Model file for the job. Use its own axes, mm. Face numbers are marked on the shaded views. A direction names the side the tool comes from. Coordinates: 2 decimals unless noted, no trailing zeros. Order: outer loops, then holes, each group sorted by start corner. A loop starts at its lowest first (then second) coordinate and runs counter-clockwise, first axis right, second up. Notation, with made-up numbers: (67.5, -27.5) -> (77.5, -27.5) arc R20 ccw to (77.5, -1.5) -> close; hole circle Ø9 at (60, 20.25). An arc over 180 degrees is marked (long way). Use CSV: the item, a comma, the result in double quotes. Start each with the question number.
(1) Cut at C-C on z = -51.5. Write the cut outline in (x, y).
(2) Pull direction Y, two halves, no side cores. Call the marked faces 1, 2, 3 and 4: pulls with the +Y half, pulls with the -Y half, needs draft (parallel to the pull), parting line crosses it, or undercut.
(3) Cut at D-D on y = 64.5. Write the cut outline in (x, z).
(4) Tool access for the marked faces 5 and 6: list every direction of +Z, -Z, +X, -X, +Y, -Y with a clear straight run to the whole face (end or side of a thin tool).
(5) Pin check, flat tips, straight feed: pin 1 Ø1.5 at (x, y) = (198, 21.5) entering from +Z; pin 2 Ø5 at (x, y) = (171.5, 54.5) entering from +Z; pin 3 Ø1.5 at (x, y) = (57, 48) entering from -Z. Stop position of each tip, or through.
(6) Cut at B-B on y = 50. Give the number of separate pieces and of enclosed holes in the cut face, plus the area to 3 significant figures.
(7) Probe L1, parallel to Y at x = 168, z = -37; L2, parallel to X at y = 78.5, z = -75.5; L3, parallel to Y at x = 9, z = -64.5. List the from-to ranges inside material, lowest first.
Autodesk Inventor part; units mm, degrees
ref_plane "YZ Plane" through (0, 0, 0) normal (1, 0, 0) x (0, 1, 0)
ref_plane "XZ Plane" through (0, 0, 0) normal (0, 1, 0) x (-1, 0, 0)
ref_plane "XY Plane" through (0, 0, 0) normal (0, 0, 1) x (1, 0, 0)
sketch "Sketch1" plane through (0, 0, 0) normal (0, 0, 1) x (1, 0, 0)
  line L0 (0, 0) -> (200, 0)
  line L1 (200, 0) -> (200, 90)
  line L2 (200, 90) -> (0, 90)
  line L3 (0, 90) -> (0, 0)
  dimension "d0" = 200
  dimension "d1" = 90
extrude "Extrusion1" add sketch "Sketch1" against normal blind 80
sketch "Sketch2" plane through (0, 90, 0) normal (0, 1, 0) x (1, 0, 0)
  line L0 (200, 0) -> (0, 0)
  line L1 (200, 0) -> (200, 80)
  line L2 (0, 80) -> (200, 80)
  line L3 (0, 0) -> (0, 80)
  circle A0 centre (100, 0) radius 30
  arc A1 (200, 0) -> (0, 0) centre (100, -151.6667) ccw
  dimension "d4" = 60
extrude "Extrusion2" cut sketch "Sketch2" against normal blind 100 contours L0 A0 A1 | L0 A0 | A0 L0 A1 picked at (94.9216, 15.5737)
fillet "Fillet1" radius 15 2 edges at (200, 45, 0) (0, 45, 0)
sketch "Sketch3" plane through (200, 0, -80) normal (1, 0, 0) x (0, 0, -1)
  line L0 (-80, 0) -> (-80, 90)
  line L1 (-80, 0) -> (0, 0)
  line L2 (0, 90) -> (0, 0)
  line L3 (-80, 90) -> (0, 90)
  line L4 (-12, 25) -> (-11.3, 25)
  line L5 (-10, 23.7) -> (-10, 16.3)
  line L6 (-11.3, 15) -> (-12, 15)
  line L7 (-13.3, 16.3) -> (-13.3, 23.7)
  arc A0 (-12, 25) -> (-13.3, 23.7) centre (-12, 23.7) ccw
  arc A1 (-10, 23.7) -> (-11.3, 25) centre (-11.3, 23.7) ccw
  arc A2 (-11.3, 15) -> (-10, 16.3) centre (-11.3, 16.3) ccw
  arc A3 (-13.3, 16.3) -> (-12, 15) centre (-12, 16.3) ccw
  point P0 (-10, 15)
  point P1 (-10, 25)
  point P2 (-13.3, 15)
  point P3 (-11.65, 15)
  dimension "d8" = 3.3
  dimension "d9" = 10
  dimension "d10" = 1.3
  dimension "d11" = 10
  dimension "d12" = 15
fillet "Fillet3" radius 10 10 edges at (7.0077, 0, -12.9892) (0, 0, -52.8413) (192.9923, 0, -12.9892) (200, 0, -52.8413) (100, 0, -30) (192.9923, 90, -12.9892) (200, 90, -52.8413) (7.0077, 90, -12.9892) (0, 90, -52.8413) (100, 90, -30)
shell "Shell2" thickness 5 removed faces 1 at (130, 30, -80)
extrude "Extrusion4" cut sketch "Sketch3" against normal blind 100 contours L4 A1 L5 A2 L6 A3 L7 A0
fillet "Fillet4" radius 1 16 edges at (200, 24.6192, -67.0808) (200, 25, -68.35) (200, 24.6192, -69.6192) (200, 20, -70) (200, 15.3808, -69.6192) (200, 15, -68.35) (200, 15.3808, -67.0808) (200, 20, -66.7) (195, 15.3808, -67.0808) (195, 15, -68.35) (195, 15.3808, -69.6192) (195, 20, -70) (195, 24.6192, -69.6192) (195, 25, -68.35) (195, 24.6192, -67.0808) (195, 20, -66.7)
sketch "Sketch6" plane through (200, 10, -25.6826) normal (1, 0, 0) x (0, 0, -1)
  line L0 (0, 70) -> (54.3174, 70)
  line L1 (0, 0) -> (0, 70)
  line L2 (54.3174, 0) -> (0, 0)
  line L3 (54.3174, 70) -> (54.3174, 0)
  arc A0 (42.3174, 16) -> (40.0174, 13.7) centre (42.3174, 13.7) ccw
  line L4 (43.0174, 16) -> (42.3174, 16)
  arc A1 (45.3174, 13.7) -> (43.0174, 16) centre (43.0174, 13.7) ccw
  line L5 (45.3174, 6.3) -> (45.3174, 13.7)
  arc A2 (43.0174, 4) -> (45.3174, 6.3) centre (43.0174, 6.3) ccw
  line L6 (42.3174, 4) -> (43.0174, 4)
  arc A3 (40.0174, 6.3) -> (42.3174, 4) centre (42.3174, 6.3) ccw
  line L7 (40.0174, 13.7) -> (40.0174, 6.3)
  line L8 (44.3174, 42.5) -> (34.3174, 42.5)
  line L9 (34.3174, 42.5) -> (34.3174, 27.5)
  line L10 (34.3174, 27.5) -> (44.3174, 27.5)
  line L11 (44.3174, 27.5) -> (44.3174, 42.5)
  point P0 (-25.6826, -10)
  point P1 (44.3174, 35)
  point P2 (54.3174, 35)
  dimension "d32" = 10
  dimension "d33" = 15
  dimension "d34" = 10
extrude "Extrusion7" cut sketch "Sketch6" against normal blind 5 contours L11 L10 L9 L8
sketch "Sketch7" plane through (0, 10, -80) normal (-1, 0, 0) x (0, 0, 1)
  line L0 (0, 70) -> (54.3174, 70)
  line L1 (0, 0) -> (0, 70)
  line L2 (54.3174, 0) -> (0, 0)
  line L3 (54.3174, 70) -> (54.3174, 0)
  line L4 (10, 42.5) -> (20, 42.5)
  line L5 (20, 42.5) -> (20, 27.5)
  line L6 (20, 27.5) -> (10, 27.5)
  line L7 (10, 27.5) -> (10, 42.5)
  point P0 (80, -10)
  point P1 (10, 35)
  point P2 (0, 35)
  dimension "d37" = 10
  dimension "d38" = 15
  dimension "d39" = 10
extrude "Extrusion8" cut sketch "Sketch7" against normal blind 5 contours L4 L5 L6 L7
fillet "Fillet5" radius 2.5 12 edges at (195, 45, -60) (195, 52.5, -65) (195, 37.5, -65) (200, 45, -60) (200, 37.5, -65) (200, 52.5, -65) (0, 45, -60) (5, 45, -60) (5, 52.5, -65) (0, 52.5, -65) (0, 37.5, -65) (5, 37.5, -65)
properties part number "BatPackCase_3DPrint"
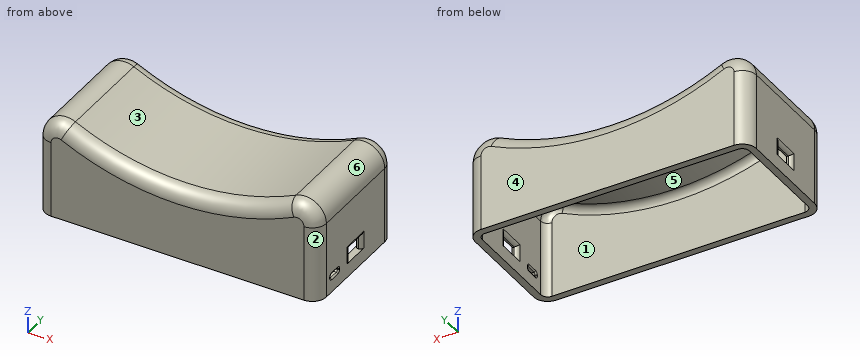
Outcome:
1,outline,"(0, 10) arc R10 ccw to (10, 0) -> (190, 0) arc R10 ccw to (200, 10) -> (200, 80) arc R10 ccw to (190, 90) -> (10, 90) arc R10 ccw to (0, 80) -> close; hole (5, 10) arc R5 ccw to (10, 5) -> (190, 5) arc R5 ccw to (195, 10) -> (195, 80) arc R5 ccw to (190, 85) -> (10, 85) arc R5 ccw to (5, 80) -> close"
2,face 1,"undercut"
2,face 2,"pulls with the -Y half"
2,face 3,"needs draft"
2,face 4,"pulls with the +Y half"
3,outline,"(0, -80) -> (5, -80) -> (5, -25.68) arc R10 cw to (19.32, -16.66) arc R186.67 ccw to (180.68, -16.66) arc R10 cw to (195, -25.68) -> (195, -80) -> (200, -80) -> (200, -25.68) arc R15 ccw to (178.52, -12.16) arc R181.67 cw to (21.48, -12.16) arc R15 ccw to (0, -25.68) -> close"
4,face 5,"-Z"
4,face 6,"+Z, +Y, -Y"
5,pin 1,"z = -17.03"
5,pin 2,"z = -14.25"
5,pin 3,"z = -30.16"
6,separate pieces,"3"
6,enclosed holes,"0"
6,area,"1,510 mm2"
7,L1,"0 to 5, 85 to 90"
7,L2,"0 to 5, 195 to 200"
7,L3,"0.05 to 5.1, 84.9 to 89.95"
